from build123d import *

# Parameters (mm, degrees)
Y_KSEKLIK_EKSTR_ZYON1_DEPTH = 2
Y_KSEKLIK_EKSTR_ZYON2_DEPTH = 2.6
IZIM3_W                     = 18
IZIM3_H                     = 13
KES_EKSTR_ZYON1_DEPTH       = 12


with BuildPart() as part:
    # Çizim1 → Yükseklik-Ekstrüzyon1 (new body)
    with BuildSketch(Plane.XY):
        with BuildLine():
            Line((-13.5, 12.5), (13.5, 12.5))
            ThreePointArc((13.5, 12.5), (15.621320344, 11.621320344), (16.5, 9.5))
            Line((16.5, 9.5), (16.5, -9.5))
            ThreePointArc((16.5, -9.5), (15.621320344, -11.621320344), (13.5, -12.5))
            Line((13.5, -12.5), (-13.5, -12.5))
            ThreePointArc((-13.5, -12.5), (-15.621320344, -11.621320344), (-16.5, -9.5))
            Line((-16.5, -9.5), (-16.5, 9.5))
            ThreePointArc((-16.5, 9.5), (-15.621320344, 11.621320344), (-13.5, 12.5))
        make_face()
    extrude(amount=Y_KSEKLIK_EKSTR_ZYON1_DEPTH)

    # Çizim2 → Yükseklik-Ekstrüzyon2 (add)
    with BuildSketch(Plane.XY.offset(2)):
        with BuildLine():
            Line((-11.5, 10.5), (11.5, 10.5))
            ThreePointArc((11.5, 10.5), (12.914213562, 9.914213562), (13.5, 8.5))
            Line((13.5, 8.5), (13.5, -8.5))
            ThreePointArc((13.5, -8.5), (12.914213562, -9.914213562), (11.5, -10.5))
            Line((11.5, -10.5), (-11.5, -10.5))
            ThreePointArc((-11.5, -10.5), (-12.914213562, -9.914213562), (-13.5, -8.5))
            Line((-13.5, -8.5), (-13.5, 8.5))
            ThreePointArc((-13.5, 8.5), (-12.914213562, 9.914213562), (-11.5, 10.5))
        make_face()
        with BuildLine():
            Line((-9.5, 8.5), (9.5, 8.5))
            ThreePointArc((9.5, 8.5), (10.914213562, 7.914213562), (11.5, 6.5))
            Line((11.5, 6.5), (11.5, -6.5))
            ThreePointArc((11.5, -6.5), (10.914213562, -7.914213562), (9.5, -8.5))
            Line((9.5, -8.5), (-9.5, -8.5))
            ThreePointArc((-9.5, -8.5), (-10.914213562, -7.914213562), (-11.5, -6.5))
            Line((-11.5, -6.5), (-11.5, 6.5))
            ThreePointArc((-11.5, 6.5), (-10.914213562, 7.914213562), (-9.5, 8.5))
        make_face(mode=Mode.SUBTRACT)
    extrude(amount=Y_KSEKLIK_EKSTR_ZYON2_DEPTH)

    # Çizim3 → Kes-Ekstrüzyon1 (cut)
    with BuildSketch(Plane.XY.offset(2)):
        Rectangle(IZIM3_W, IZIM3_H)
    extrude(amount=-KES_EKSTR_ZYON1_DEPTH, mode=Mode.SUBTRACT)


solid = part.part
The listing builds one solid part. Answer for the finished solid, in the listing's coordinates (mm). A direction names the side the tool comes from. Coordinates: 2 decimals unless noted, no trailing zeros. Loops run counter-clockwise (first coordinate to the right, second up) from the corner with the lowest first, then second, coordinate; pieces in that order, holes last.
1) A tool of negligible diameter and unlimited length cuts with its end or side. For faces 5 (the face through (-9, 0, 1)), 6 (the face through (11.5, 0, 3)), 7 (the face through (12.9, 9.93, 3.28)), from which of +Z, -Z, +X, -X, +Y, -Y can it reach the whole face along a straight path? Write none if from no direction.
2) Find section B-B on y = -5.5. Write down the section's boundary in (x, z).
3) Find the intervals of material crossed by L1, parallel to Y at x = -4.5, z = 1.95; L2, parallel to Y at x = -2, z = 3.8; L3, parallel to X at y = -3.5, z = 1.8, in increasing order.
4) Determine the mould class of faces 1 (the face through (-11.5, 0, 3)), 2 (the face through (-10.93, 7.9, 3.28)), 3 (the face through (-16.5, 0, 1)), 4 (the face through (0, -11, 2)) for opening direction X: pulls with the +X half, pulls with the -X half, needs draft (parallel to the pull), parting line crosses it, or undercut.
5) Flat-ended cylindrical pins translate along their axes: pin 1 Ø1.3 at (x, z) = (0, 3.5) entering from +Y; pin 2 Ø1 at (x, z) = (-12.5, 3.5) entering from -Y; pin 3 Ø2 at (x, y) = (12, 10) entering from -Z; pin 4 Ø0.8 at (y, z) = (1.5, 3) entering from +X. Find the tip coordinate at first contact, or state that the pin passes through.
6) Find section D-D on y = 10. Write down the section's boundary in (x, z), then the cut area to 3 significant figures.
7) Find section A-A on x = -0.5. Write down the section's boundary in (y, z).
8) Find section C-C on z = 4.05. Write down the section's boundary in (x, y).
Values:
1. face 5: +Z, -Z
1. face 6: +Z
1. face 7: +Z, +X, +Y
2. outline: (-16.5, 0) - (-9, 0) - (-9, 2) - (-11.5, 2) - (-11.5, 4.6) - (-13.5, 4.6) - (-13.5, 2) - (-16.5, 2) - close; (9, 0) - (16.5, 0) - (16.5, 2) - (13.5, 2) - (13.5, 4.6) - (11.5, 4.6) - (11.5, 2) - (9, 2) - close
3. L1: y = -12.5 to -6.5, 6.5 to 12.5
3. L2: y = -10.5 to -8.5, 8.5 to 10.5
3. L3: x = -16.5 to -9, 9 to 16.5
4. face 1: undercut
4. face 2: undercut
4. face 3: pulls with the -X half
4. face 4: needs draft
5. pin 1: stops at y = 10.5
5. pin 2: stops at y = -10.44
5. pin 3: stops at z = 0
5. pin 4: stops at x = 13.5
6. outline: (-16.46, 0) - (16.46, 0) - (16.46, 2) - (12.82, 2) - (12.82, 4.6) - (-12.82, 4.6) - (-12.82, 2) - (-16.46, 2) - close
6. area: 133 mm2
7. outline: (-12.5, 0) - (-6.5, 0) - (-6.5, 2) - (-8.5, 2) - (-8.5, 4.6) - (-10.5, 4.6) - (-10.5, 2) - (-12.5, 2) - close; (6.5, 0) - (12.5, 0) - (12.5, 2) - (10.5, 2) - (10.5, 4.6) - (8.5, 4.6) - (8.5, 2) - (6.5, 2) - close
8. outline: (-13.5, -8.5) arc R2 ccw to (-11.5, -10.5) - (11.5, -10.5) arc R2 ccw to (13.5, -8.5) - (13.5, 8.5) arc R2 ccw to (11.5, 10.5) - (-11.5, 10.5) arc R2 ccw to (-13.5, 8.5) - close; hole (-11.5, -6.5) arc R2 ccw to (-9.5, -8.5) - (9.5, -8.5) arc R2 ccw to (11.5, -6.5) - (11.5, 6.5) arc R2 ccw to (9.5, 8.5) - (-9.5, 8.5) arc R2 ccw to (-11.5, 6.5) - close
